Model file for the job. Use its own axes, mm. A direction names the side the tool comes from. Coordinates: 2 decimals unless noted, no trailing zeros. Write each loop counter-clockwise with the first axis right and the second up, starting at its lowest first coordinate (ties: lowest second). Pieces come first, ordered by that corner, then holes. Notation, with made-up numbers: (81, -31) -> (86, -31) arc R19 ccw to (86, -26) -> close; hole circle Ø7 at (-16.75, 23.5). An arc over 180 degrees is marked (long way). Answer as a JSON object with one key per item and string values. Group by question number.
Autodesk Inventor part; units mm, degrees
ref_plane "YZ Plane" through (0, 0, 0) normal (1, 0, 0) x (0, 1, 0)
ref_plane "XZ Plane" through (0, 0, 0) normal (0, 1, 0) x (-1, 0, 0)
ref_plane "XY Plane" through (0, 0, 0) normal (0, 0, 1) x (1, 0, 0)
sketch "Sketch1" plane through (0, 0, 0) normal (0, 0, 1) x (1, 0, 0)
  arc A0 (-5.5118, -5.25) -> (-5.5118, 21.75) centre (-8.0118, 8.25) ccw construction
  circle A1 centre (-7.8118, 8.25) radius 10 construction
  circle A2 centre (-7.8118, 8.25) radius 12.15 construction
  line L0 (-5.5118, -8.25) -> (-5.5118, -5.25) construction
  line L1 (7.4882, -8.25) -> (-5.5118, -8.25) construction
  line L2 (11.0118, -4.7265) -> (7.4882, -8.25) construction
  line L3 (11.0118, -4.7265) -> (11.0118, 21.2265) construction
  line L4 (11.0118, 21.2265) -> (7.4882, 24.75) construction
  line L5 (7.4882, 24.75) -> (-5.5118, 24.75) construction
  line L6 (-5.5118, 24.75) -> (-5.5118, 21.75) construction
  arc A3 (-5.5118, -5.25) -> (-5.5118, 21.75) centre (-8.0118, 8.25) ccw construction
  line L7 (5.7178, 24.75) -> (38.7178, 24.75) construction
  circle A4 centre (-26.8118, 8.25) radius 1.45
  circle A5 centre (4.6882, -4.25) radius 1.45
  arc A6 (-22.4732, 11.4188) -> (-22.4732, 5.0812) centre (-7.8118, 8.25) ccw
  line L8 (-22.4732, 5.0812) -> (-3.2253, -6.0316) construction
  arc A7 (-3.2253, -6.0316) -> (2.2632, -2.8628) centre (-7.8118, 8.25) ccw
  line L9 (2.2632, 19.3628) -> (2.2632, -2.8628) construction
  arc A8 (2.2632, 19.3628) -> (-3.2253, 22.5316) centre (-7.8118, 8.25) ccw
  line L10 (-22.4732, 11.4188) -> (-3.2253, 22.5316) construction
  line L11 (-32.9624, -8.8) -> (-32.9624, 25.3)
  line L12 (-32.9624, 25.3) -> (-29.2731, 25.3)
  line L13 (-29.2731, 25.3) -> (-24.8618, 29.7113)
  line L14 (-24.8618, 29.7113) -> (-24.8618, 33.4006)
  line L15 (-24.8618, 33.4006) -> (9.2382, 33.4006)
  line L16 (9.2382, 33.4006) -> (9.2382, 29.7113)
  line L17 (9.2382, 29.7113) -> (13.6496, 25.3)
  line L18 (13.6496, 25.3) -> (17.3389, 25.3)
  line L19 (17.3389, 25.3) -> (17.3389, -8.8)
  line L20 (17.3389, -8.8) -> (13.6496, -8.8)
  line L21 (13.6496, -8.8) -> (9.2382, -13.2113)
  line L22 (9.2382, -13.2113) -> (9.2382, -16.9006)
  line L23 (9.2382, -16.9006) -> (-24.8618, -16.9006)
  line L24 (-24.8618, -16.9006) -> (-24.8618, -13.2113)
  line L25 (-24.8618, -13.2113) -> (-29.2731, -8.8)
  line L26 (-29.2731, -8.8) -> (-32.9624, -8.8)
  circle A9 centre (4.6882, 20.75) radius 1.45
  line L27 (-21.7254, -4.75) -> (-31.0589, 8.25)
  line L28 (-31.0589, 8.25) -> (-20.8118, 21.25)
  circle A10 centre (-7.8118, 8.25) radius 12.5 construction
  circle A11 centre (4.6882, -4.25) radius 2.45
  circle A12 centre (4.6882, 20.75) radius 2.45
  circle A13 centre (-26.8118, 8.25) radius 2.45
  circle A14 centre (-7.8118, 8.25) radius 10
  circle A15 centre (-7.8118, 8.25) radius 10
  circle A16 centre (-7.8118, 8.25) radius 10
  circle A17 centre (-7.8118, 8.25) radius 12.25
  line L29 (-20.8118, 21.25) -> (8.1382, 24.6257)
  line L30 (8.1382, 24.6257) -> (8.1382, -8.1099)
  line L31 (8.1382, -8.1099) -> (-21.7254, -4.75)
  circle A18 centre (4.6882, -4.25) radius 3.45 construction
  circle A19 centre (4.6882, 20.75) radius 3.45 construction
  circle A20 centre (-26.8118, 8.25) radius 3.45 construction
  dimension "d12" = 13
  dimension "d14" = 13
  dimension "d15" = 13
  dimension "d16" = 0
  dimension "d17" = 4.9
  dimension "d18" = 4.9
  dimension "d19" = 4.9
  dimension "d25" = 24.5
  dimension "d32" = 1
  dimension "d33" = 1
  dimension "d35" = 1
extrude "Extrusion1" add sketch "Sketch1" along normal blind 4 contours L27 L28 L29 L30 L31
sketch "Sketch3" plane through (0, 0, 0) normal (0, 0, -1) x (-1, 0, 0)
  circle A0 centre (-4.6882, 20.75) radius 1.45
  circle A1 centre (26.8118, 8.25) radius 1.45
  circle A2 centre (-4.6882, -4.25) radius 1.45
  circle A3 centre (7.8118, 8.25) radius 14
  line L0 (1.437, 26.1707) -> (-0.0466, 24.25)
  line L1 (1.437, 25.85) -> (1.437, 26.1707)
  line L2 (7.7704, 25.85) -> (1.437, 25.85)
  line L3 (7.7704, 32.85) -> (7.7704, 25.85)
  line L4 (15.1593, 24.25) -> (7.7704, 32.85)
  line L5 (15.1593, 24.25) -> (23.8118, 24.25)
  line L6 (23.8118, 24.25) -> (30.5959, 9.0658)
  arc A4 (30.5959, 7.4342) -> (30.5959, 9.0658) centre (28.7698, 8.25) ccw
  line L7 (30.5959, 7.4342) -> (23.8118, -7.75)
  line L8 (23.8118, -7.75) -> (15.1593, -7.75)
  line L9 (15.1593, -7.75) -> (7.7704, -16.35)
  line L10 (7.7704, -9.35) -> (7.7704, -16.35)
  line L11 (1.437, -9.35) -> (7.7704, -9.35)
  line L12 (1.437, -9.6707) -> (1.437, -9.35)
  line L13 (1.437, -9.6707) -> (-0.0466, -7.75)
  line L14 (-0.0466, -7.75) -> (-8.1882, -7.75)
  line L15 (-8.1882, -7.75) -> (-10.9318, -5.0065)
  line L16 (-10.9318, -5.0065) -> (-10.9318, 21.5065)
  line L17 (-10.9318, 21.5065) -> (-8.1882, 24.25)
  line L18 (-8.1882, 24.25) -> (-0.0466, 24.25)
  point P0 (0, 0)
fillet "Fillet1" radius 2 5 edges at (-31.0589, 8.25, 2) (-20.8118, 21.25, 2) (-21.7254, -4.75, 2) (8.1382, 24.6257, 2) (8.1382, -8.1099, 2)
sketch "Sketch5" plane through (-21.3259, 20.5977, 0) normal (-0.7853545, 0.6190463, 0) x (0, 0, 1)
  circle A0 centre (1.8492, -5.6115) radius 1.45
  point P0 (0, -2.9748)
  dimension "d21" = 2.9
extrude "Extrusion3" cut sketch "Sketch5" against normal blind 10
sketch "Sketch6" plane through (0, 0, 4) normal (0, 0, 1) x (1, 0, 0)
  arc A0 (-19.9868, 21.3462) -> (-21.3259, 20.5977) centre (-19.7552, 19.3596) ccw
  line L0 (-21.3259, 20.5977) -> (-30.1272, 9.432)
  arc A1 (-30.1272, 9.432) -> (-30.1811, 7.0274) centre (-28.5565, 8.1939) ccw
  line L1 (-30.1811, 7.0274) -> (-22.2435, -4.0283)
  arc A2 (-22.2435, -4.0283) -> (-20.8425, -4.8493) centre (-20.6189, -2.8619) ccw
  circle A3 centre (-26.8118, 8.25) radius 2.45
  circle A4 centre (4.6882, 20.75) radius 2.45
  circle A5 centre (4.6882, -4.25) radius 2.45
  circle A6 centre (-7.8118, 8.25) radius 12.25
  line L2 (-20.8425, -4.8493) -> (5.9146, -7.8597)
  line L3 (8.1382, -5.8723) -> (8.1382, 22.3789)
  line L4 (5.9066, 24.3654) -> (-19.9868, 21.3462)
  arc A7 (5.9146, -7.8597) -> (8.1382, -5.8723) centre (6.1382, -5.8723) ccw
  arc A8 (8.1382, 22.3789) -> (5.9066, 24.3654) centre (6.1382, 22.3789) ccw
  point P0 (0, 0)
extrude "Extrusion4" add sketch "Sketch6" along normal blind 6 contours L4 A8 L3 A7 L2 A2 L1 A1 L0 A0 | A3 | A4 | A5
sketch "Sketch7" plane through (8.1382, -5.9842, 0) normal (1, 0, 0) x (0, 0, -1)
  spline S0 degree 3 poles (-20.3248, 15.4894) (-20.4822, 15.4894) (-20.6498, 15.4578) (-20.9577, 15.3301) (-21.098, 15.234) (-21.3195, 15.0125) (-21.4156, 14.8722) (-21.5433, 14.5643) (-21.5748, 14.3967) (-21.5748, 14.082) (-21.5433, 13.9144) (-21.4156, 13.6065) (-21.3195, 13.4662) (-21.098, 13.2447) (-20.9577, 13.1486) (-20.6498, 13.0209) (-20.4822, 12.9894) (-20.1675, 12.9894) (-19.9999, 13.0209) (-19.692, 13.1486) (-19.5517, 13.2447) (-19.3302, 13.4662) (-19.2341, 13.6065) (-19.1064, 13.9144) (-19.0748, 14.082) (-19.0748, 14.3967) (-19.1064, 14.5643) (-19.2341, 14.8722) (-19.3302, 15.0125) (-19.5517, 15.234) (-19.692, 15.3301) (-19.9999, 15.4578) (-20.1675, 15.4894) (-20.3248, 15.4894) knots 0 0 0 0 0.047214 0.047214 0.094427 0.094427 0.141639 0.141639 0.18885 0.18885 0.236062 0.236062 0.283273 0.283273 0.330487 0.330487 0.3777 0.3777 0.424914 0.424914 0.472128 0.472128 0.519339 0.519339 0.56655 0.56655 0.613762 0.613762 0.660973 0.660973 0.708187 0.708187 0.755401 0.755401 0.755401 0.755401
  circle A0 centre (-14.6316, 14.3711) radius 1.45
  circle A1 centre (-7.8169, 14.3711) radius 1.45
  point P0 (0, 5.9842)
  point P1 (-20.3248, 15.4894)
  dimension "d28" = 2.9
  dimension "d29" = 2.9
extrude "Extrusion5" cut sketch "Sketch7" against normal blind 16 contours A0 | A1
properties part number "cellSTORM_inverted_objectiveadapter"
(1) Pin check, flat tips, straight feed: pin 1 (12 mm diameter, centred on x = -7, y = 9, fed in from +Z); pin 2 (8 mm diameter, centred on x = -25, y = 17, fed in from +Z); pin 3 (4.5 mm diameter, centred on x = -26.81, y = 8.25, fed in from -Z); pin 4 (1.5 mm diameter, centred on x = -7.5, z = 4, fed in from -Y). Stop position of each tip, or through.
(2) Cut at C-C on z = 1.25. List the corners of the cut face in (x, y), plus the area to 3 significant figures.
(3) Cut at A-A on x = -15. List the corners of the cut face in (y, z), plus the area to 3 significant figures.
(4) Cut at D-D on x = -27.5. List the corners of the cut face in (y, z) (3 decimals), plus the area to 3 significant figures.
(5) Pull direction X, two halves, no side cores. Call faces 4 (the face through (-27, 8, 4)), 5 (the face through (-30.556, 8.257, 2.028)), 6 (the face through (-20, 5, 10)), 7 (the face through (-25.681, 10.424, 1.972)): released by +X, released by -X, zero draft, split by the parting line, or undercut.
(6) Cut at B-B on y = 0.5. List the corners of the cut face in (x, z).
(7) Wall check: probe 1 along Y at (x, z) = (5, 3.5); probe 2 along X at (y, z) = (15, 1.5); probe 3 along X at (y, z) = (15.5, 2.75). Give the ranges that are in metal, low to high.
(8) 3-axis set-ups, long thin cutter, end or side, ignore diameter. For faces 1 (the face through (8.138, 8, 5)), 2 (the face through (6.95, 21.69, 1.97)), 3 (the face through (6.263, 8.451, 9.265)): which of +Z, -Z, +X, -X, +Y, -Y reach the whole face in a straight line?
Results found:
{
 "1": {"pin 1": "passes through", "pin 2": "stops at z = 10", "pin 3": "stops at z = 4", "pin 4": "stops at y = -6.43"},
 "2": {"outline": "(-30.18, 7.03) -> (-22.24, -4.03) arc R2 ccw to (-20.84, -4.85) -> (5.91, -7.86) arc R2 ccw to (8.14, -5.87) -> (8.14, 22.38) arc R2 ccw to (5.91, 24.37) -> (-19.99, 21.35) arc R2 ccw to (-21.33, 20.6) -> (-23.98, 17.23) -> (-18.98, 13.28) arc R12.25 cw (long way) to (-19.84, 10.6) -> (-25.62, 15.15) -> (-30.13, 9.43) arc R2 ccw to start; hole circle Ø4.9 at (-26.81, 8.25); hole circle Ø4.9 at (4.69, -4.25); hole circle Ø4.9 at (4.69, 20.75)", "area": "442 mm²"},
 "3": {"outline": "(-5.51, 0) -> (-1.67, 0) -> (-1.67, 10) -> (-5.51, 10) -> close; (18.17, 0) -> (21.93, 0) -> (21.93, 10) -> (18.17, 10) -> close", "area": "76.0 mm²"},
 "4": {"outline": "(3.293, 0) -> (5.899, 0) -> (5.899, 4) -> (10.601, 4) -> (10.601, 0) -> (12.765, 0) -> (12.765, 10) -> (3.293, 10) -> close", "area": "75.9 mm²"},
 "5": {"face 4": "undercut", "face 5": "released by -X", "face 6": "zero draft", "face 7": "undercut"},
 "6": {"outline": "(-25.49, 0) -> (-17.3, 0) -> (-17.3, 10) -> (-25.49, 10) -> close; (1.68, 0) -> (8.14, 0) -> (8.14, 10) -> (1.68, 10) -> close"},
 "7": {"probe 1": "y = -7.76 to -6.68, -1.82 to 18.32, 23.18 to 24.26", "probe 2": "x = -25.74 to -25.56, -21.02 to -18.03, 2.41 to 8.14", "probe 3": "x = -22.09 to -17.69, 2.06 to 8.14"},
 "8": {"face 1": "+Z, -Z, +X, +Y, -Y", "face 2": "-Z", "face 3": "+X"}
}
